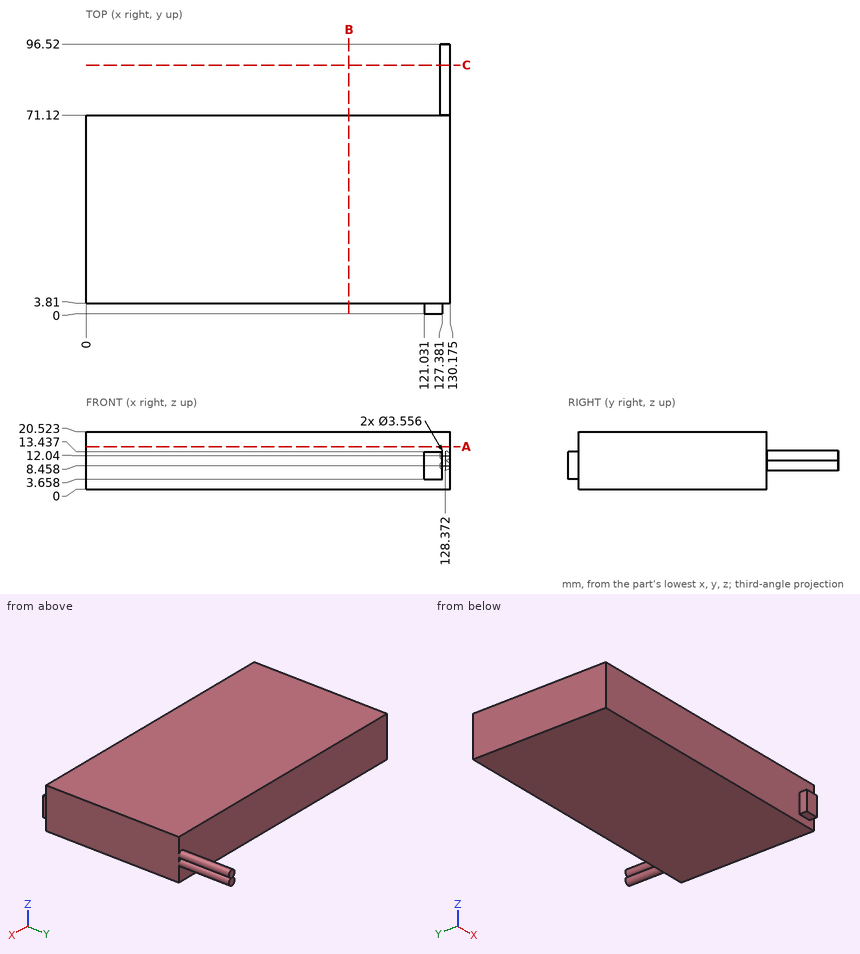
Can you work these out from the drawing? Everything is in mm from the part's minimum corner. Coordinates: 2 decimals unless noted, no trailing zeros. Loops run counter-clockwise (first coordinate to the right, second up) from the corner with the lowest first, then second, coordinate; pieces in that order, holes last. Notation, with made-up numbers: (12.5, 80.25) -> (25.5, 80.25) arc R7 ccw to (25.5, 91.25) -> close; hole circle Ø5 at (70, -9.5). An arc over 180 degrees is marked (long way). Return JSON: item names as keys, results as strings.
1) If we section it at A-A, the plane z = 15.25: Write out the boundary of the cut face in (x, y) (1 decimal), then the cut area to 3 significant figures.
Results below:
{"outline": "(0, 3.8) -> (130.2, 3.8) -> (130.2, 71.1) -> (0, 71.1) -> close", "area": "8,760 mm²"}
2) If we section it at B-B, the plane x = 94: Write out the boundary of the cut face in (y, z), then the cut area to 3 significant figures.
Results below:
{"outline": "(3.81, 0) -> (71.12, 0) -> (71.12, 20.52) -> (3.81, 20.52) -> close", "area": "1,380 mm²"}
3) I need wall thicknesses on line 1 (Y direction, x = 42.5, z = 12); line 2 (X direction, y = 87, z = 7) (1 decimal); line 3 (X direction, y = 86, z = 12.5) (1 decimal). Which ranges of each line are inside material? Lowest first, please. Write a range as from..to.
Results below:
{"line 1": "3.81..71.12", "line 2": "127.4..129.4", "line 3": "126.7..130.1"}
4) If we section it at C-C, the plane y = 89: Write out the boundary of the cut face in (x, z).
Results below:
{"outline": "circle Ø3.56 at (128.37, 8.46); circle Ø3.56 at (128.37, 12.04)"}
5) Will these pins go through, and if not, where does the flat tip stop? pin 1 (2 mm diameter, centred on x = 64.5, z = 15.5, fed in from +Y); pin 2 (1 mm diameter, centred on x = 71.5, y = 64.5, fed in from -Z); pin 3 (6 mm diameter, centred on x = 42, z = 9.5, fed in from -Y); pin 4 (1.9 mm diameter, centred on x = 123.5, y = 2.5, fed in from +Z).
Results below:
{"pin 1": "y = 71.12", "pin 2": "z = 0", "pin 3": "y = 3.81", "pin 4": "z = 13.44"}
